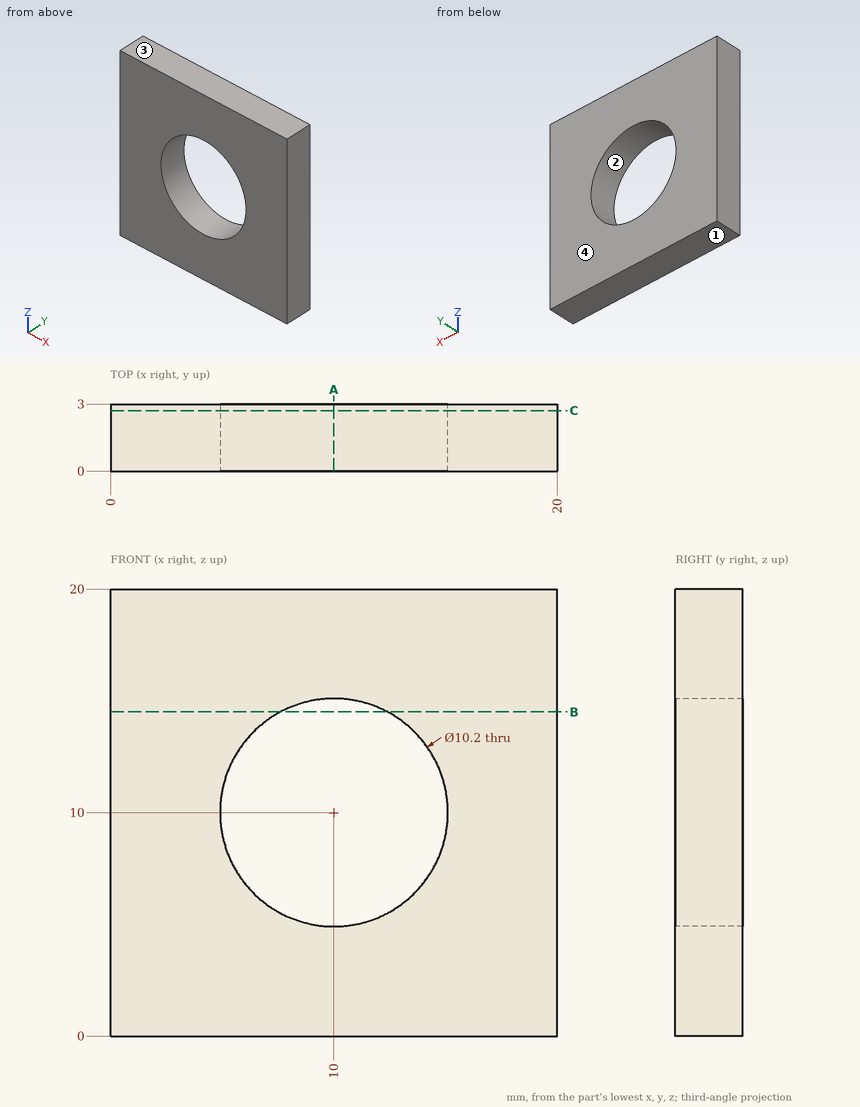
Print and shaded views of the part. All mm, measured from the part's lowest x, y and z. Coordinates: 2 decimals unless noted, no trailing zeros. Order: outer loops, then holes, each group sorted by start corner. A loop starts at its lowest first (then second) coordinate and runs counter-clockwise, first axis right, second up. Notation, with made-up numbers: M 51,81 L 92,81 A5 ccw 92,90 Z; hole C 44,31 d1. An arc over 180 degrees is marked long. Write each question's results on one line, items separated by ' | '. Start each with the question number.
Q1. Cut at B-B (z = 14.5). List the corners of the cut face in (x, y).
Q2. Pull direction Z, two halves, no side cores. Call the marked faces 1, 2, 3 and 4: +Z half, -Z half, draft (parallel to the pull), parting line (faces both ways), or undercut.
Q3. Drill centre lines: probe 1 along Z at (x, y) = (10, 1.25); probe 2 along X at (y, z) = (1.5, 14.25); probe 3 along X at (y, z) = (1.2, 13). Where is each one in solid material? Low to high. Write a range as from..to.
Q4. Cut at A-A (x = 10). List the corners of the cut face in (y, z).
Q5. Cut at C-C (y = 2.7). List the corners of the cut face in (x, z), then the cut area to 3 significant figures.
Found:
1) outline: M 0,0 L 7.6,0 L 7.6,3 L 0,3 Z; M 12.4,0 L 20,0 L 20,3 L 12.4,3 Z
2) face 1: -Z half | face 2: undercut | face 3: +Z half | face 4: draft
3) probe 1: 0..4.9, 15.1..20 | probe 2: 0..7.18, 12.82..20 | probe 3: 0..5.88, 14.12..20
4) outline: M 0,0 L 3,0 L 3,4.9 L 0,4.9 Z; M 0,15.1 L 3,15.1 L 3,20 L 0,20 Z
5) outline: M 0,0 L 20,0 L 20,20 L 0,20 Z; hole C 10,10 d10.2 | area: 318 mm²
